```python
from build123d import *


with BuildPart() as part:
    # Эскиз1 → Повернуть1 (revolve)
    with BuildSketch(Plane.XY, mode=Mode.PRIVATE) as revolve_1_sk:
        Polygon((-9, 5), (9, 5), (9, 8), (2.8, 8), (2.8, 12), (9, 12), (9, 17.8), (6.3, 17.8), (6.3, 13.8), (1.3, 13.8), (-1.3, 13.8), (-6.3, 13.8), (-6.3, 17.8), (-9, 17.8), (-9, 12), (-2.8, 12), (-2.8, 8), (-9, 8), align=None)
    revolve(revolve_1_sk.sketch.rotate(Axis((0, 0, 0), (-1, 0, 0)), 90), axis=Axis((0, 0, 0), (-1, 0, 0)))

    # Эскиз2 → Повернуть2 (revolve)
    with BuildSketch(Plane.XY, mode=Mode.PRIVATE) as revolve_2_sk:
        with BuildLine():
            Line((-1.3, 13.3), (1.3, 13.3))
            ThreePointArc((1.3, 13.3), (0.798778164, 13.993411613), (0, 14.3))
            ThreePointArc((0, 14.3), (-0.798778164, 13.993411613), (-1.3, 13.3))
        make_face()
    revolve(revolve_2_sk.sketch.rotate(Axis((0, 0, 0), (1, 0, 0)), 270), axis=Axis((0, 0, 0), (1, 0, 0)))


solid = part.part
```
Could you check a few things on this model? Use its own coordinates, in mm. A direction names the side the tool comes from. Round coordinates to 2 decimals unless told otherwise and drop trailing zeros. Write each loop counter-clockwise with the first axis right and the second up, starting at its lowest first coordinate (ties: lowest second). Pieces come first, ordered by that corner, then holes. Notation, with made-up numbers: M -28,-23.5 L -3,-23.5 A17 cw -3,-5.5 Z; hole C 87,-38.75 d4. An arc over 180 degrees is marked long. Write each question's results on one line, items separated by ' | '. Start each with the question number.
1. I need wall thicknesses on L1, parallel to Y at x = 5.5, z = 0; L2, parallel to X at y = 0.5, z = 16; L3, parallel to X at y = -7.5, z = 12. Which ranges of each line are inside material? Lowest first, please. Write a range as from..to.
2. Imagine slicing it at C-C on x = -1.5. List the corners of the cut face in (y, z) for me.
3. Imagine slicing it at A-A on x = 5. List the corners of the cut face in (y, z) for me.
4. Thinking about a two-plate mould opening in Z: for faces 5 (the face through (5.943, -3.604, -11.446)), 6 (the face through (9, -0.1, 5.2)), 7 (the face through (7.63, -12.03, 13.12)), which applies, +Z half, -Z half, draft (parallel to the pull), parting line (faces both ways), or undercut?
5. I'm going to push flat-ended pins straight in: pin 1 Ø6 at (x, y) = (1, 12) entering from -Z; pin 2 Ø1 at (x, z) = (-0.5, -8.5) entering from +Y; pin 3 Ø1 at (x, y) = (3, 0) entering from +Z. Where does each tip first touch, or does it pass through?
6. On a 3-axis mill with a long thin cutter (end or side, diameter ignored), from which of +Z, -Z, +X, -X, +Y, -Y can I reach the whole of each face in a straight line? I mean faces 1 (the face through (-6.3, 13.1, 5.2)), 2 (the face through (2.8, 8, 2)), 3 (the face through (-9, 5.2, 0.1)), 4 (the face through (-5.94, 7.81, 1.73)). Say none if no direction works.
7. Imagine slicing it at B-B on y = -15. List the corners of the cut face in (x, z) for me, and give its area (4 significant figures).
Result sheet:
1) L1: y = -13.8..-12, -8..-5, 5..8, 12..13.8 | L2: x = -9..-6.3, 6.3..9 | L3: x = -9..-6.3, -0.55..0.55, 6.3..9
2) outline: C 0,0 d27.6; hole C 0,0 d10
3) outline: C 0,0 d27.6; C 0,0 d16; hole C 0,0 d24; hole C 0,0 d10
4) face 5: undercut | face 6: draft | face 7: parting line
5) pin 1: stops at z = -10.99 | pin 2: stops at y = 11.76 | pin 3: stops at z = 13.8
6) face 1: none | face 2: +X | face 3: +Z, -Z, -X, +Y, -Y | face 4: -X
7) outline: M -9,-9.58 L -6.3,-9.58 L -6.3,9.58 L -9,9.58 Z; M 6.3,-9.58 L 9,-9.58 L 9,9.58 L 6.3,9.58 Z | area: 103.5 mm^2
